from build123d import *

# Parameters (mm, degrees)
SKETCH1_W           = 100.17
SKETCH1_H           = 9.87
BOSS_EXTRUDE1_DEPTH = 3.175
SKETCH2_R           = 1.415
CUT_EXTRUDE1_DEPTH  = 4.175
SKETCH3_R           = 1.415
CUT_EXTRUDE2_DEPTH  = 4.175


with BuildPart() as part:
    # Sketch1 → Boss-Extrude1 (new body)
    with BuildSketch(Plane.XY):
        Rectangle(SKETCH1_W, SKETCH1_H)
    extrude(amount=BOSS_EXTRUDE1_DEPTH)

    # Sketch2 → Cut-Extrude1 (cut, through all)
    with BuildSketch(Plane.XY.offset(3.175)):
        with Locations((-44.696699141, -0.453300859)):
            Circle(SKETCH2_R)
        with Locations((44.696699141, -0.453300859)):
            Circle(SKETCH2_R)
    extrude(amount=-CUT_EXTRUDE1_DEPTH, mode=Mode.SUBTRACT)

    # Sketch3 → Cut-Extrude2 (cut, through all)
    with BuildSketch(Plane.XY.offset(3.175)):
        with Locations((0, -0.453300859)):
            Circle(SKETCH3_R)
    extrude(amount=-CUT_EXTRUDE2_DEPTH, mode=Mode.SUBTRACT)


solid = part.part
CAD build for the part. Positions are in the model's coordinates, mm. Round coordinates to 2 decimals unless told otherwise and drop trailing zeros. Order: outer loops, then holes, each group sorted by start corner. A loop starts at its lowest first (then second) coordinate and runs counter-clockwise, first axis right, second up. Notation, with made-up numbers: (16.5, 77) -> (74.5, 77) arc R31 cw to (74.5, 108) -> close; hole circle Ø1 at (1.25, 3). An arc over 180 degrees is marked (long way). Write item = value, one per line. Start each with the question number.
(1) Pin check, flat tip, straight feed: P1, Ø2.5, axis at x = 0, y = -0.45, coming from the -Z side. Stop position of the tip, or through.
(2) Probe line 1 (X direction, y = -1.25, z = 2.65) (3 decimals); line 2 (Y direction, x = 0, z = 2) (3 decimals). List the from-to ranges inside material, lowest first. Write a range as [from, to].
(3) Cut at A-A, the plane x = 0. List the corners of the cut face in (y, z) (3 decimals), then the cut area to 3 significant figures.
(4) Pull direction X, two halves, no side cores. Call faces 1 (the cylindrical face through (-46.11, -0.39, 1.61)), 2 (the flat face through (50.085, 0, 2)), 3 (the flat face through (-1, 1, 3.175)): released by +X, released by -X, zero draft, split by the parting line, or undercut.
(5) Cut at B-B, the plane z = 1.65. List the corners of the cut face in (x, y) (3 decimals), then the cut area to 3 significant figures.
Model answer:
q1.P1 = through
q2.line_1 = [-50.085, -45.866], [-43.527, -1.169], [1.169, 43.527], [45.866, 50.085]
q2.line_2 = [-4.935, -1.868], [0.962, 4.935]
q3.outline = (-4.935, 0) -> (-1.868, 0) -> (-1.868, 3.175) -> (-4.935, 3.175) -> close; (0.962, 0) -> (4.935, 0) -> (4.935, 3.175) -> (0.962, 3.175) -> close
q3.area = 22.4 mm2
q4.face_1 = undercut
q4.face_2 = released by +X
q4.face_3 = zero draft
q5.outline = (-50.085, -4.935) -> (50.085, -4.935) -> (50.085, 4.935) -> (-50.085, 4.935) -> close; hole circle Ø2.83 at (-44.697, -0.453); hole circle Ø2.83 at (0, -0.453); hole circle Ø2.83 at (44.697, -0.453)
q5.area = 970 mm2
